Geometry check sheet. Reference: the model listing, model coordinates, mm. Round coordinates to 2 decimals unless told otherwise and drop trailing zeros. Write each loop counter-clockwise with the first axis right and the second up, starting at its lowest first coordinate (ties: lowest second). Pieces come first, ordered by that corner, then holes. Notation, with made-up numbers: M 54.5,74 L 65.5,74 A20 ccw 65.5,95 Z; hole C -21,-22 d3. An arc over 180 degrees is marked long. One line per item, written item: value. Start each with the question number.
1. Depth check by flat-ended pin: P1, Ø4, axis at x = -23.3, y = 6.25, coming from the -Z side. Enter the tip coordinate at first touch or a pass-through.
2. Scan lines: probe 1 along X at (y, z) = (6.5, 1.3); probe 2 along X at (y, z) = (4, 0.15); probe 3 along Y at (x, z) = (20, 1.55). Record each from-to range of solid material in increasing order. Write a range as [from, to].
3. Section check C-C (x = 24). Record the boundary of the cut face in (y, z).
4. Section check A-A (x = -39). Record the boundary of the cut face in (y, z), and give its area (3 significant figures).
5. Section check B-B (z = 1.55). Record the boundary of the cut face in (x, y) (3 decimals), and give its area (3 significant figures).
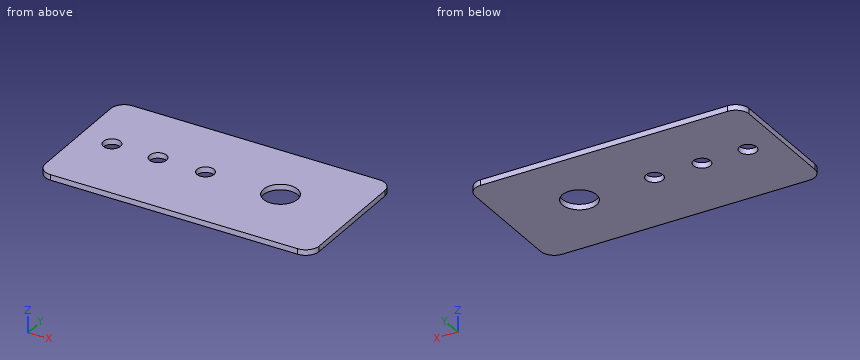
from build123d import *

# Parameters (mm, degrees)
F0_W     = 101.6
F0_H     = 50.8
F1_DEPTH = 2.032
F2_R     = 5
F4_D     = 6.35
F6_D     = 12.7


with BuildPart() as f1:
    # F0 (on Top) → F1 (new body)
    with BuildSketch(Plane.XY):
        with Locations((-1.363633, 4.882393)):
            Rectangle(F0_W, F0_H)
    extrude(amount=F1_DEPTH)

    # F2
    f2_edges = [f1.edges().sort_by_distance(p)[0] for p in [
        (-52.163633, 30.282393, 1.016),
        (49.436367, 30.282393, 1.016),
        (-52.163633, -20.517607, 1.016),
        (49.436367, -20.517607, 1.016),
    ]]
    fillet(f2_edges, radius=F2_R)

    # F4 (through all)
    with Locations(Plane.XY.offset(2.032)):
        with Locations((-40.383019, 6.245364), (-23.299415, 6.245364), (-5.693044, 6.245364)):
            Hole(F4_D / 2)

    # F6 (through all)
    with Locations(Plane.XY.offset(2.032)):
        with Locations((22.099847, 6.288829)):
            Hole(F6_D / 2)


solid = f1.part
Result sheet:
1. P1: passes through
2. probe 1: x = [-52.16, -43.55], [-37.22, -26.46], [-20.13, -8.86], [-2.53, 15.75], [28.45, 49.44]
2. probe 2: x = [-52.16, -42.63], [-38.14, -25.54], [-21.05, -7.94], [-3.45, 16.18], [28.02, 49.44]
2. probe 3: y = [-20.52, 0.3], [12.28, 30.28]
3. outline: M -20.52,0 L 0.23,0 L 0.23,2.03 L -20.52,2.03 Z; M 12.35,0 L 30.28,0 L 30.28,2.03 L 12.35,2.03 Z
4. outline: M -20.52,0 L 3.39,0 L 3.39,2.03 L -20.52,2.03 Z; M 9.1,0 L 30.28,0 L 30.28,2.03 L 9.1,2.03 Z
4. area: 91.6 mm2
5. outline: M -52.164,-15.518 A5 ccw -47.164,-20.518 L 44.436,-20.518 A5 ccw 49.436,-15.518 L 49.436,25.282 A5 ccw 44.436,30.282 L -47.164,30.282 A5 ccw -52.164,25.282 Z; hole C -40.383,6.245 d6.35; hole C -23.299,6.245 d6.35; hole C -5.693,6.245 d6.35; hole C 22.1,6.289 d12.7
5. area: 4,920 mm2
